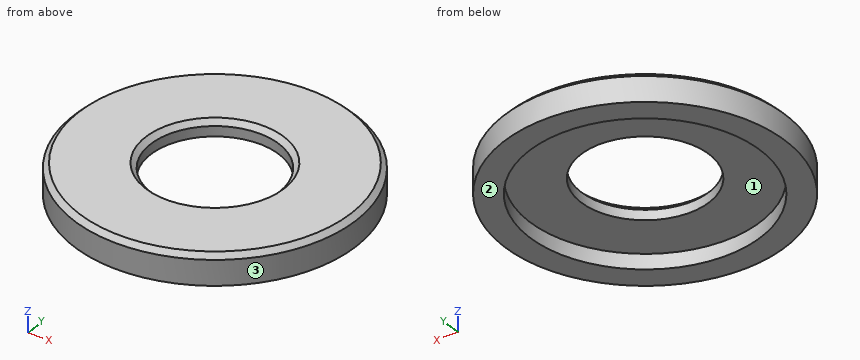
```python
from build123d import *

# Parameters (mm, degrees)
F0_R     = 28
F0_R_2   = 23
F1_DEPTH = 6
F2_DEPTH = 3
F3_R     = 12.75
F4_DEPTH = 6.001
F5_SIZE  = 1


with BuildPart() as f1:
    # F0 (on Top) → F1 (new body)
    with BuildSketch(Plane.XY):
        Circle(F0_R)
        Circle(F0_R_2, mode=Mode.SUBTRACT)
        Circle(F0_R_2)
    extrude(amount=F1_DEPTH)

    # F0 (on Top) → F2 (cut)
    with BuildSketch(Plane.XY):
        Circle(F0_R_2)
    extrude(amount=F2_DEPTH, mode=Mode.SUBTRACT)

    # F3 (on face) → F4 (cut, through all)
    with BuildSketch(Plane.XY.offset(6)):
        Circle(F3_R)
    extrude(amount=-F4_DEPTH, mode=Mode.SUBTRACT)

    # F5
    f5_edges = [f1.edges().sort_by_distance(p)[0] for p in [
        (-12.75, 0, 6),
        (-28, 0, 6),
    ]]
    chamfer(f5_edges, length=F5_SIZE)


solid = f1.part
```
Build history of the part. All positions in model axes, mm. Face numbers are marked on the shaded views. Give positions to 0.01 mm unless a question says otherwise; leave off trailing zeros. Order: outer loops, then holes, each group sorted by start corner. A loop starts at its lowest first (then second) coordinate and runs counter-clockwise, first axis right, second up. Notation, with made-up numbers: M 43,-21.75 L 93,-21.75 A16 cw 93,-8.75 Z; hole C 37.25,39.5 d7. An arc over 180 degrees is marked long. Write item = value, one per line. Start each with the question number.
(1) Pin check, flat tips, straight feed: pin 1 Ø3 at (x, y) = (19.5, -2) entering from -Z; pin 2 Ø1.5 at (y, z) = (-9, 1.5) entering from -X; pin 3 Ø20.5 at (x, y) = (0, 0) entering from -Z; pin 4 Ø5 at (x, y) = (-20, -8) entering from -Z. Stop position of each tip, or through.
(2) Slice it at C-C on z = 1.65. Write the cut outline in (x, y), plus the area to 3 significant figures.
(3) Slice it at A-A on y = 0. Write the cut outline in (x, z).
(4) Probe L1, parallel to Y at x = 0, z = 1.7; L2, parallel to Y at x = 0, z = 3.4; L3, parallel to Z at x = 18, y = 6. List the from-to ranges inside material, lowest first. Write a range as [from, to].
(5) Two-plate mould, pull along X, no slides. Class the marked faces 1, 2 and 3: released by +X, released by -X, zero draft, split by the parting line, or undercut.
Responses:
q1.pin_1 = 3
q1.pin_2 = -26.76
q1.pin_3 = through
q1.pin_4 = 0
q2.outline = C 0,0 d56; hole C 0,0 d46
q2.area = 801 mm2
q3.outline = M -28,0 L -23,0 L -23,3 L -12.75,3 L -12.75,5 L -13.75,6 L -27,6 L -28,5 Z; M 12.75,3 L 23,3 L 23,0 L 28,0 L 28,5 L 27,6 L 13.75,6 L 12.75,5 Z
q4.L1 = [-28, -23], [23, 28]
q4.L2 = [-28, -12.75], [12.75, 28]
q4.L3 = [3, 6]
q5.face_1 = undercut
q5.face_2 = zero draft
q5.face_3 = split by the parting line
